from build123d import *

# Parameters (mm, degrees)
SKETCH1_W          = 203.2
SKETCH1_H          = 152.4
EXTRUDE1_DEPTH     = 25.4
CUT_EXTRUDE1_DEPTH = 19.05
CUT_EXTRUDE1_DRAFT = -6
FILLET1_R          = 6.35


with BuildPart() as part:
    # Sketch1 → Extrude1 (new body)
    with BuildSketch(Plane.XY):
        with Locations((101.6, 76.2)):
            Rectangle(SKETCH1_W, SKETCH1_H)
    extrude(amount=EXTRUDE1_DEPTH)


with BuildPart() as cut_extrude1_tool:
    # Sketch2 → Cut-Extrude1 (with draft: the straight prism first)
    with BuildSketch(Plane.XY.offset(25.4)):
        Polygon((19.319910515, 132.568680089), (19.319910515, 14.376286353), (75.688590604, 14.376286353), (75.688590604, 51.652348993), (116.904399702, 51.652348993), (116.904399702, 14.376286353), (186.607606264, 14.376286353), (186.607606264, 132.568680089), (116.904399702, 132.568680089), (116.904399702, 74.684712901), (75.688590604, 74.684712901), (75.688590604, 132.568680089), align=None)
    extrude(amount=-CUT_EXTRUDE1_DEPTH)
    # Cut-Extrude1: the draft: its side faces are tilted about the plane it starts from
    cut_extrude1_sides = [cut_extrude1_tool.faces().sort_by_distance(p)[0] for p in [
        (19.319910515, 73.472483221, 15.875),
        (47.504250559, 14.376286353, 15.875),
        (75.688590604, 33.014317673, 15.875),
        (96.296495153, 51.652348993, 15.875),
        (116.904399702, 33.014317673, 15.875),
        (151.756002983, 14.376286353, 15.875),
        (186.607606264, 73.472483221, 15.875),
        (151.756002983, 132.568680089, 15.875),
        (116.904399702, 103.626696495, 15.875),
        (96.296495153, 74.684712901, 15.875),
        (75.688590604, 103.626696495, 15.875),
        (47.504250559, 132.568680089, 15.875),
    ]]
    draft(cut_extrude1_sides, Plane.XY.offset(25.4), CUT_EXTRUDE1_DRAFT)


with BuildPart() as part_1:
    add(part.part)

    # Cut-Extrude1: cut by cut_extrude1_tool
    add(cut_extrude1_tool.part, mode=Mode.SUBTRACT)

    # Fillet1
    fillet1_edges = [part_1.edges().sort_by_distance(p)[0] for p in [
        (20.321028355, 131.567562249, 15.875),
        (20.321028355, 15.377404194, 15.875),
        (74.687472763, 15.377404194, 15.875),
        (74.687472763, 52.653466834, 15.875),
        (117.905517543, 15.377404194, 15.875),
        (185.606488423, 15.377404194, 15.875),
        (185.606488423, 131.567562249, 15.875),
        (117.905517543, 131.567562249, 15.875),
        (117.905517543, 73.68359506, 15.875),
        (74.687472763, 73.68359506, 15.875),
        (74.687472763, 131.567562249, 15.875),
    ]]
    fillet(fillet1_edges, radius=FILLET1_R)


solid = part_1.part
Check sheet for the modelled part. Datum: model origin and axes. Units: mm. A direction names the side the tool comes from. Give positions to 0.01 mm unless a question says otherwise; leave off trailing zeros. Write each loop counter-clockwise with the first axis right and the second up, starting at its lowest first coordinate (ties: lowest second). Pieces come first, ordered by that corner, then holes. Notation, with made-up numbers: M 56,-12 L 89,-12 A17 cw 89,2 Z; hole C 69.25,60 d2. An arc over 180 degrees is marked long. Use one line per item in the form item = value.
(1) Material ranges on line 1 along X through (y, z) = (88, 6.5); line 2 along X through (y, z) = (80.5, 23.25); line 3 along Z through (x, y) = (182, 23), recorded low to high.
Answer block:
line_1 = 0 to 21.31, 73.7 to 118.89, 184.62 to 203.2
line_2 = 0 to 19.55, 75.47 to 117.12, 186.38 to 203.2
line_3 = 0 to 6.35
(2) Section check B-B on x = 175.5. Record the boundary of the cut face in (y, z).
Answer block:
outline = M 0,0 L 152.4,0 L 152.4,25.4 L 132.57,25.4 L 130.57,6.35 L 16.38,6.35 L 14.38,25.4 L 0,25.4 Z
(3) Tool access check on faces 1 (the flat face through (100, 152.4, 13)), 2 (the flat face through (74.7, 102.3, 16)). Record the directions out of +Z, -Z, +X, -X, +Y, -Y that give a thin tool (end or side, any length) a straight path to the whole face; none if there is none.
Answer block:
face_1 = +Z, -Z, +X, -X, +Y
face_2 = +Z
(4) Draft check along X on faces 3 (the flat face through (100, 77, 25.4)), 4 (the flat face through (0, 75, 13)), 5 (the flat face through (99.18, 52.64, 16.01)). Enter one of: pulls with the +X half, pulls with the -X half, needs draft (parallel to the pull), parting line crosses it, or undercut.
Answer block:
face_3 = needs draft
face_4 = pulls with the -X half
face_5 = undercut
(5) Section check A-A on y = 67. Record the boundary of the cut face in (x, z), plus the area to 3 significant figures.
Answer block:
outline = M 0,0 L 203.2,0 L 203.2,25.4 L 186.61,25.4 L 184.61,6.35 L 21.32,6.35 L 19.32,25.4 L 0,25.4 Z
area = 2,010 mm2
(6) Section check C-C on y = 39. Record the boundary of the cut face in (x, z).
Answer block:
outline = M 0,0 L 203.2,0 L 203.2,25.4 L 186.61,25.4 L 184.61,6.35 L 118.91,6.35 L 116.9,25.4 L 75.69,25.4 L 73.69,6.35 L 21.32,6.35 L 19.32,25.4 L 0,25.4 Z
